Drawing for the job (mm, zero at the part's lowest x, y, z). Give positions to 0.01 mm unless a question says otherwise; leave off trailing zeros. Loops run counter-clockwise (first coordinate to the right, second up) from the corner with the lowest first, then second, coordinate; pieces in that order, holes last. Notation, with made-up numbers: M 46.25,35.25 L 70.25,35.25 A26 cw 70.25,74.25 Z; hole C -14.75,-3 d10. An arc over 180 degrees is marked long. Use CSV: the item, a comma, the result in double quotes. Start each with the question number.
(1) Slice it at B-B on y = 125. List the corners of the cut face in (x, z).
(2) Slice it at D-D on y = 18. List the corners of the cut face in (x, z), and give its area (4 significant figures).
(3) Flat gauge pins, fed straight in: P1, Ø1.5, axis at x = 2, y = 28, coming from the -Z side; P2, Ø1.5, axis at x = 2.5, y = 66, coming from the -Z side; P3, Ø12, axis at y = 39, z = 21, coming from the -X side; P4, Ø1, axis at x = 2.5, y = 74, coming from the -Z side. Where does each tip first touch, or does it go through?
(4) Wall check: line 1 along Z through (x, y) = (4.65, 138.5); line 2 along Y through (x, z) = (0.8, 3.5); line 3 along Y through (x, z) = (3.1, 18.5). Give the ranges that are in metal, low to high. Write a range as from..to.
(5) Slice it at C-C on x = 3. List the corners of the cut face in (y, z), and give its area (3 significant figures).
(6) Slice it at A-A on z = 9.5. List the corners of the cut face in (x, y).
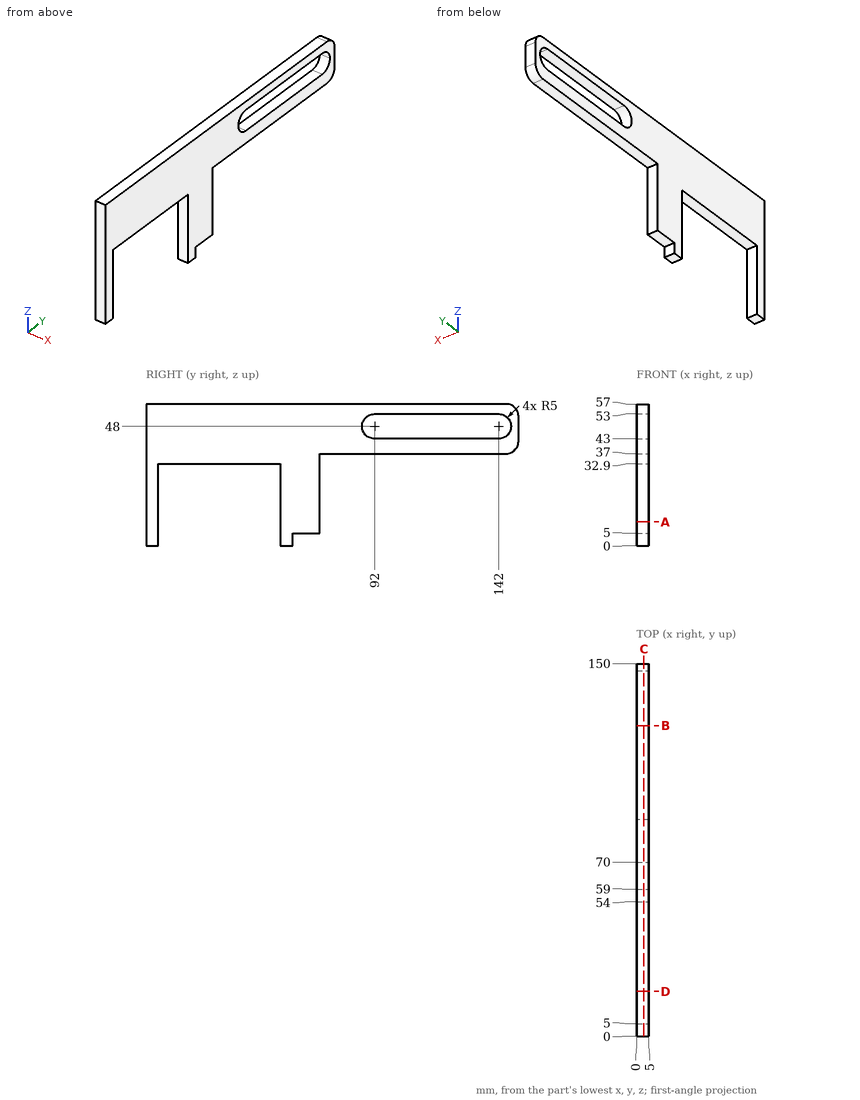
Reply:
1,outline,"M 0,37 L 5,37 L 5,43 L 0,43 Z; M 0,53 L 5,53 L 5,57 L 0,57 Z"
2,outline,"M 0,32.9 L 5,32.9 L 5,57 L 0,57 Z"
2,area,"120.5 mm^2"
3,P1,"stops at z = 32.9"
3,P2,"stops at z = 5"
3,P3,"passes through"
3,P4,"stops at z = 37"
4,line 1,"z = 37..43, 53..57"
4,line 2,"y = 0..5, 54..59"
4,line 3,"y = 0..5, 54..70"
5,outline,"M 0,0 L 5,0 L 5,32.9 L 54,32.9 L 54,0 L 59,0 L 59,5 L 70,5 L 70,37 L 145,37 A5 ccw 150,42 L 150,52 A5 ccw 145,57 L 0,57 Z; hole M 92,43 L 142,43 A5 ccw 142,53 L 92,53 A5 ccw Z"
5,area,"3,330 mm^2"
6,outline,"M 0,0 L 5,0 L 5,5 L 0,5 Z; M 0,54 L 5,54 L 5,70 L 0,70 Z"
